Geometry check sheet. Reference: the model listing, model coordinates, mm. A direction names the side the tool comes from. Give positions to 0.01 mm unless a question says otherwise; leave off trailing zeros. Write each loop counter-clockwise with the first axis right and the second up, starting at its lowest first coordinate (ties: lowest second). Pieces come first, ordered by that corner, then holes.
(1) Mould release check, pull along X, two halves, no side actions. Record for faces 1 (the flat face through (0, 19, 67.5)), 2 (the flat face through (-20, 19, 1)), 3 (the cylindrical face through (-2.89, 20.78, -3.77)), 4 (the flat face through (20, 19, 1)): +X half, -X half, draft (parallel to the pull), parting line (faces both ways), or undercut.
(2) Cross-section at C-C (z = 0). Record the boundary of the cut face in (x, y).
(3) Cross-section at B-B (y = 10.25). Record the boundary of the cut face in (x, z), and give its area (3 significant figures).
(4) Cross-section at A-A (x = 8.5). Record the boundary of the cut face in (y, z).
(5) Cross-section at D-D (x = 0). Record the boundary of the cut face in (y, z).
(6) Thickness scan on line 1 along X through (y, z) = (19.95, 0); line 2 along Z through (x, y) = (-2.5, 14.25); line 3 along X through (y, z) = (11.5, 0). Record the ranges inside material, lowest first.
(7) Depth check by flat-ended pin: P1, Ø8, axis at x = 3.5, z = 26, coming from the -Y side; P2, Ø0.8, axis at x = -4.5, y = 14, coming from the -Z side; P3, Ø2, axis at x = -0.5, z = 0.5, coming from the +Y side. Enter the tip coordinate at first touch or a pass-through.
(8) Tool access check on faces 5 (the flat face through (0, 14, 37.5)), 6 (the flat face through (0, 14, -35.5)), 7 (the cylindrical face through (-2, 13, 0)), 8 (the flat face through (0, 14, -37.5)), 9 (the cylindrical face through (-2.343, 7.395, -3.055)). Record the directions out of +Z, -Z, +X, -X, +Y, -Y that give a thin tool (end or side, any length) a straight path to the whole face; none if there is none.
```python
from build123d import *

# Parameters (mm, degrees)
SKETCH1_R           = 3.85
BOSS_EXTRUDE1_DEPTH = 15
SKETCH2_W           = 40
SKETCH2_H           = 135
BOSS_EXTRUDE3_DEPTH = 8
SKETCH3_W           = 40
SKETCH3_H           = 2
BOSS_EXTRUDE4_DEPTH = 2.5
SKETCH4_R           = 4.75
CUT_EXTRUDE1_DEPTH  = 4.5
SKETCH5_R           = 2
CUT_EXTRUDE2_DEPTH  = 11


with BuildPart() as part:
    # Sketch1 → Boss-Extrude1 (new body)
    with BuildSketch(Plane(origin=(0, 0, 0), x_dir=(1, 0, 0), z_dir=(0, 1, 0))):
        with Locations(Location((0, 0, 0), (0, 0, 270))):
            Circle(SKETCH1_R)
    extrude(amount=BOSS_EXTRUDE1_DEPTH)

    # Sketch2 → Boss-Extrude3 (add)
    with BuildSketch(Plane(origin=(0, 15, 0), x_dir=(1, 0, 0), z_dir=(0, 1, 0))):
        Rectangle(SKETCH2_W, SKETCH2_H)
    extrude(amount=BOSS_EXTRUDE3_DEPTH)

    # Sketch3 → Boss-Extrude4 (add)
    with BuildSketch(Plane.XZ.offset(-15)):
        with Locations((0, -36.5)):
            Rectangle(SKETCH3_W, SKETCH3_H)
        with Locations((0, 36.5)):
            Rectangle(SKETCH3_W, SKETCH3_H)
    extrude(amount=BOSS_EXTRUDE4_DEPTH)

    # Sketch4 → Cut-Extrude1 (cut)
    with BuildSketch(Plane(origin=(0, 23, 0), x_dir=(1, 0, 0), z_dir=(0, 1, 0))):
        with Locations(Location((0, 0, 0), (0, 0, 270))):
            Circle(SKETCH4_R)
    extrude(amount=-CUT_EXTRUDE1_DEPTH, mode=Mode.SUBTRACT)

    # Sketch5 → Cut-Extrude2 (cut)
    with BuildSketch(Plane(origin=(0, 18.5, 0), x_dir=(1, 0, 0), z_dir=(0, 1, 0))):
        with Locations(Location((0, 0, 0), (0, 0, 270))):
            Circle(SKETCH5_R)
    extrude(amount=-CUT_EXTRUDE2_DEPTH, mode=Mode.SUBTRACT)


solid = part.part
```
Reply:
1. face 1: draft
1. face 2: -X half
1. face 3: undercut
1. face 4: +X half
2. outline: (-20, 15) - (-3.85, 15) - (-3.85, 0) - (3.85, 0) - (3.85, 15) - (20, 15) - (20, 23) - (4.75, 23) - (4.75, 18.5) - (2, 18.5) - (2, 7.5) - (-2, 7.5) - (-2, 18.5) - (-4.75, 18.5) - (-4.75, 23) - (-20, 23) - close
3. outline: circle Ø7.7 at (0, 0); hole circle Ø4 at (0, 0)
3. area: 34.0 mm2
4. outline: (12.5, -37.5) - (15, -37.5) - (15, -67.5) - (23, -67.5) - (23, 67.5) - (15, 67.5) - (15, 37.5) - (12.5, 37.5) - (12.5, 35.5) - (15, 35.5) - (15, -35.5) - (12.5, -35.5) - close
5. outline: (0, -3.85) - (15, -3.85) - (15, -35.5) - (12.5, -35.5) - (12.5, -37.5) - (15, -37.5) - (15, -67.5) - (23, -67.5) - (23, -4.75) - (18.5, -4.75) - (18.5, -2) - (7.5, -2) - (7.5, 2) - (18.5, 2) - (18.5, 4.75) - (23, 4.75) - (23, 67.5) - (15, 67.5) - (15, 37.5) - (12.5, 37.5) - (12.5, 35.5) - (15, 35.5) - (15, 3.85) - (0, 3.85) - close
6. line 1: x = -20 to -4.75, 4.75 to 20
6. line 2: z = -37.5 to -35.5, -2.93 to 2.93, 35.5 to 37.5
6. line 3: x = -3.85 to -2, 2 to 3.85
7. P1: stops at y = 15
7. P2: stops at z = -37.5
7. P3: stops at y = 7.5
8. face 5: +Z, +X, -X, -Y
8. face 6: +X, -X, -Y
8. face 7: +Y
8. face 8: -Z, +X, -X, -Y
8. face 9: -Y
